Here's the drawing with two shaded views (mm, measured from the low corner). I have some questions. A direction names the side the tool comes from. Give positions to 0.01 mm unless a question says otherwise; leave off trailing zeros. Loops run counter-clockwise (first coordinate to the right, second up) from the corner with the lowest first, then second, coordinate; pieces in that order, holes last. Notation, with made-up numbers: M -23,81 L 16,81 A19 cw 16,106 Z; hole C -18.75,-10.75 d1. An arc over 180 degrees is marked long. Use CSV: the item, a comma, the result in double quotes.
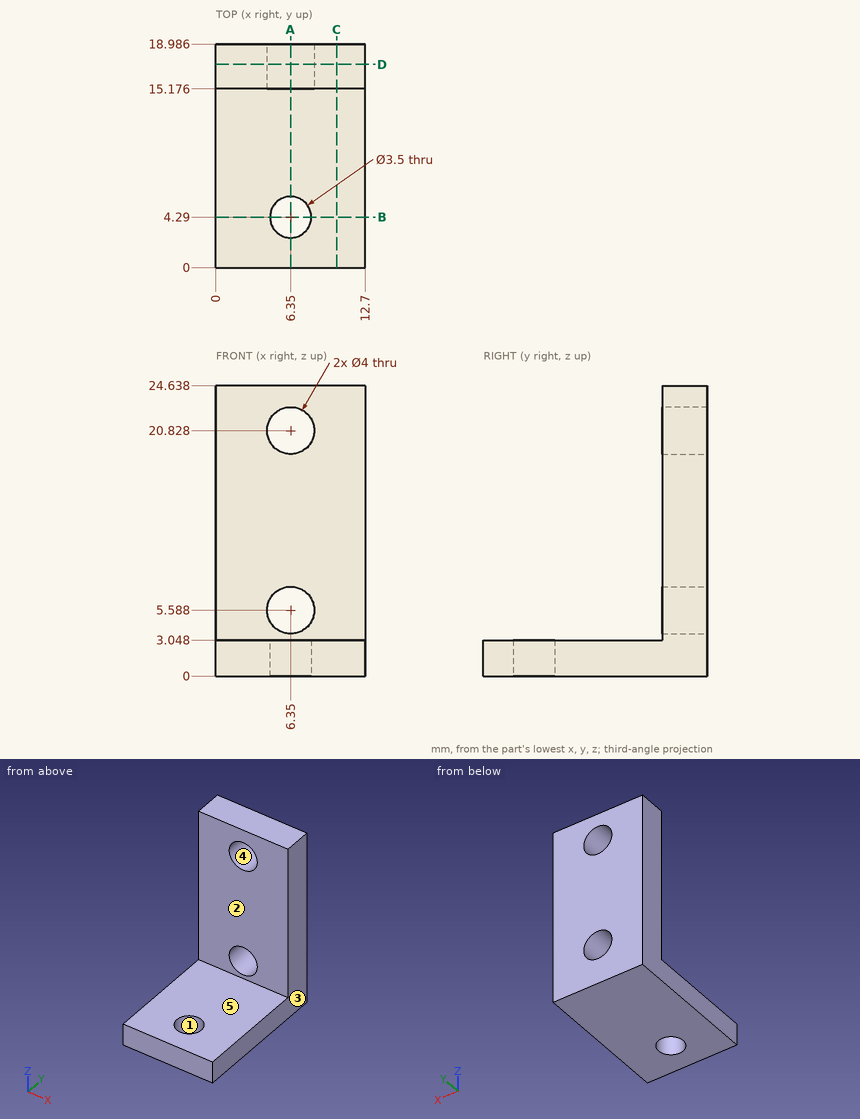
1. I want a section at C-C, the plane x = 10.25. List the corners of the cut face in (y, z) for me, then the cut area to 3 significant figures.
Outcome:
outline,"M 0,0 L 18.99,0 L 18.99,24.64 L 15.18,24.64 L 15.18,3.05 L 0,3.05 Z"
area,"140 mm2"
2. Which directions (+Z, -Z, +X, -X, +Y, -Y) give clear straight access to the entire face, cutting with the end or side of a thin tool? Please do the marked faces 1 and 2.
Outcome:
face 1,"+Z, -Z"
face 2,"+Z, +X, -X, -Y"
3. If we mould it in two halves opening along X, with no side actions, what happens to the marked faces 3, 4 and 5? For each: +X half, -X half, draft (parallel to the pull), parting line (faces both ways), or undercut.
Outcome:
face 3,"+X half"
face 4,"undercut"
face 5,"draft"
4. I want a section at A-A, the plane x = 6.35. List the corners of the cut face in (y, z) for me.
Outcome:
outline,"M 0,0 L 2.54,0 L 2.54,3.05 L 0,3.05 Z; M 6.04,0 L 18.99,0 L 18.99,3.59 L 15.18,3.59 L 15.18,3.05 L 6.04,3.05 Z; M 15.18,7.59 L 18.99,7.59 L 18.99,18.83 L 15.18,18.83 Z; M 15.18,22.83 L 18.99,22.83 L 18.99,24.64 L 15.18,24.64 Z"
5. I want a section at B-B, the plane y = 4.29. List the corners of the cut face in (x, z) for me, then the cut area to 3 significant figures.
Outcome:
outline,"M 0,0 L 4.6,0 L 4.6,3.05 L 0,3.05 Z; M 8.1,0 L 12.7,0 L 12.7,3.05 L 8.1,3.05 Z"
area,"28.0 mm2"
6. Please list where these lines run through material, in increasing order: line 1 (X direction, y = 4.29, z = 2.45); line 2 (Y direction, x = 7.25, z = 13.5); line 3 (Y direction, x = 6.35, z = 1.7).
Outcome:
line 1,"0 to 4.6, 8.1 to 12.7"
line 2,"15.18 to 18.99"
line 3,"0 to 2.54, 6.04 to 18.99"
7. I'm going to push flat-ended pins straight in: pin 1 Ø10 at (y, z) = (15, 19.5) entering from -X; pin 2 Ø10 at (y, z) = (3, 8.5) entering from -X; pin 3 Ø3 at (x, z) = (1.5, 19.5) entering from -Y. Where does each tip first touch, or does it pass through?
Outcome:
pin 1,"x = 0"
pin 2,"through"
pin 3,"y = 15.18"
8. I want a section at D-D, the plane y = 17.25. List the corners of the cut face in (x, z) for me, then the cut area to 3 significant figures.
Outcome:
outline,"M 0,0 L 12.7,0 L 12.7,24.64 L 0,24.64 Z; hole C 6.35,5.59 d4; hole C 6.35,20.83 d4"
area,"288 mm2"
